Check sheet for the modelled part. Datum: model origin and axes. Units: mm. A direction names the side the tool comes from. Round coordinates to 2 decimals unless told otherwise and drop trailing zeros. Write each loop counter-clockwise with the first axis right and the second up, starting at its lowest first coordinate (ties: lowest second). Pieces come first, ordered by that corner, then holes.
Item 1: Release check for a two-part mould opening along Y. For faces 1 (the flat face through (84, 61, 5)), 2 (the flat face through (31.31, 113.69, 3)), 3 (the flat face through (84, 120, 2)) record: +Y half, -Y half, draft (parallel to the pull), parting line (faces both ways), or undercut.
Item 2: Material ranges on line 1 (X direction, y = 115, z = 2.05); line 2 (Y direction, x = 110, z = 3.3); line 3 (Y direction, x = 140, z = 2.55), recorded low to high.
Item 3: Tool access check on faces 4 (the cylindrical face through (81.953, 5.134, 4.014)), 5 (the flat face through (84, 61, 0)). Record the directions out of +Z, -Z, +X, -X, +Y, -Y that give a thin tool (end or side, any length) a straight path to the whole face; none if there is none.
Item 4: Cross-section at A-A on x = 140. Enter the section's corners in (y, z), plus the area to 3 significant figures.
Item 5: Go/stop test with a flat-tipped pin: pin 1 Ø1.8 at (x, y) = (30, 114) entering from +Z. Record where the tip stops, or that it passes through.
from build123d import *

# Parameters (mm, degrees)
BOX_W            = 170
BOX_H            = 120
BOX_DEPTH        = 5
HOLE_D           = 3.4
HOLE_DEPTH       = 25
HOLE_CBORE_D     = 6.1
HOLE_CBORE_DEPTH = 2
SKETCH001_R      = 1.25
HOLE001_DEPTH    = 5.001
FILLET_R         = 2


with BuildPart() as part:
    # Box → Box (join)
    with BuildSketch(Plane.XY):
        with Locations((85, 60)):
            Rectangle(BOX_W, BOX_H)
    extrude(amount=BOX_DEPTH)

    # Hole
    with Locations(Plane.XY.offset(5)):
        with Locations((30, 115), (140, 115), (85, 5)):
            CounterBoreHole(HOLE_D / 2, HOLE_CBORE_D / 2, HOLE_CBORE_DEPTH, depth=HOLE_DEPTH)

    # Sketch001 (on Face5 of Hole) → Hole001 (cut, through all)
    with BuildSketch(Plane(origin=(0, 0, 0), x_dir=(1, 0, 0), z_dir=(0, 0, -1))):
        with Locations((60, -115)):
            Circle(SKETCH001_R)
        with Locations((110, -115)):
            Circle(SKETCH001_R)
    extrude(amount=-HOLE001_DEPTH, mode=Mode.SUBTRACT)

    # Fillet
    fillet_edges = [part.edges().sort_by_distance(p)[0] for p in [
        (0, 120, 2.5),
        (170, 0, 2.5),
        (0, 0, 2.5),
        (170, 120, 2.5),
    ]]
    fillet(fillet_edges, radius=FILLET_R)


solid = part.part
Response values:
1. face 1: draft
1. face 2: undercut
1. face 3: +Y half
2. line 1: x = 0 to 28.3, 31.7 to 58.75, 61.25 to 108.75, 111.25 to 138.3, 141.7 to 170
2. line 2: y = 0 to 113.75, 116.25 to 120
2. line 3: y = 0 to 113.3, 116.7 to 120
3. face 4: +Z
3. face 5: -Z, +X, -X, +Y, -Y
4. outline: (0, 0) - (113.3, 0) - (113.3, 3) - (111.95, 3) - (111.95, 5) - (0, 5) - close; (116.7, 0) - (120, 0) - (120, 5) - (118.05, 5) - (118.05, 3) - (116.7, 3) - close
4. area: 578 mm2
5. pin 1: stops at z = 3
